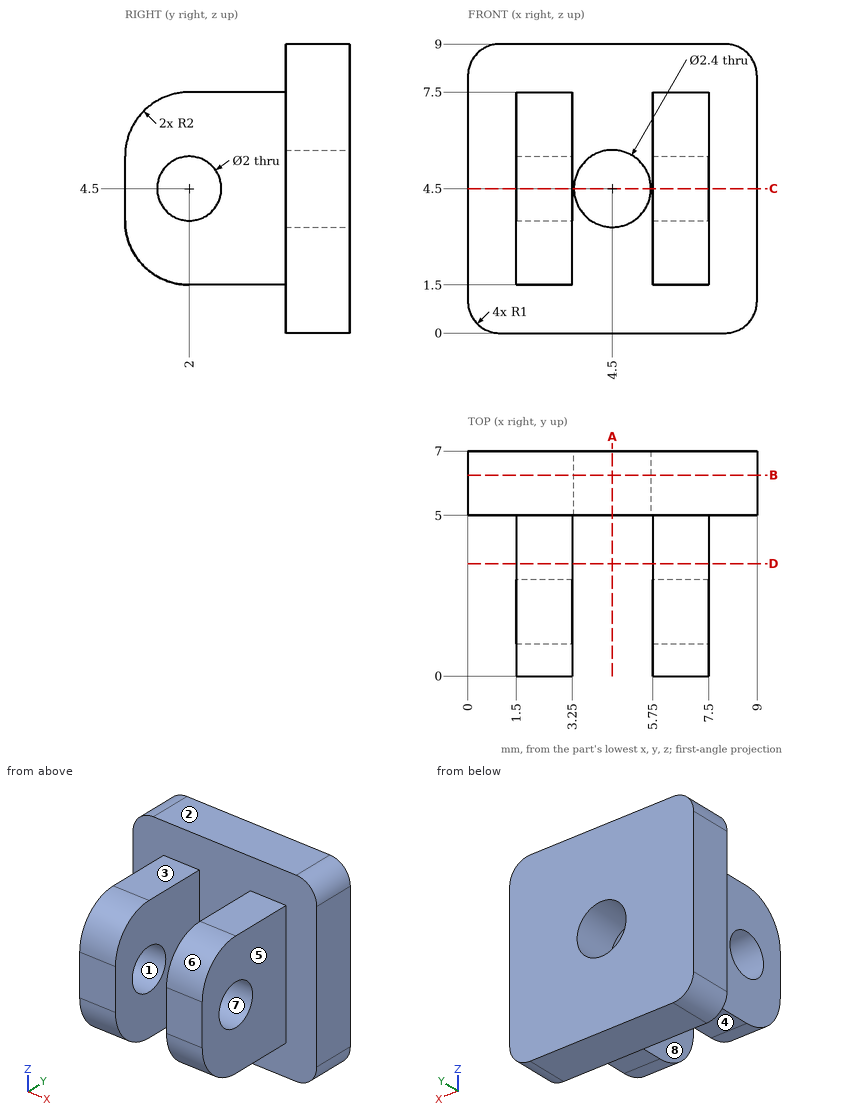
Job drawing, mm, ordinate dimensions from the low corner. One solid piece. A direction names the side the tool comes from. Coordinates: 2 decimals unless noted, no trailing zeros. Order: outer loops, then holes, each group sorted by start corner. A loop starts at its lowest first (then second) coordinate and runs counter-clockwise, first axis right, second up. Notation, with made-up numbers: (19, 21.25) -> (41, 21.25) arc R23 ccw to (41, 41.25) -> close; hole circle Ø11 at (6.25, -3). An arc over 180 degrees is marked (long way). Put each result on its own line as item: value. Start each with the question number.
(1) Pin check, flat tips, straight feed: pin 1 Ø1.9 at (x, y) = (6.5, 3) entering from +Z; pin 2 Ø2.5 at (y, z) = (3, 4) entering from +X; pin 3 Ø1.5 at (y, z) = (3, 4) entering from -X. Stop position of each tip, or through.
(2) Band-saw the part on B-B (y = 6.25). Give the cut face in (x, z).
(3) Band-saw the part on A-A (x = 4.5). Give the cut face in (y, z), then the cut area to 3 significant figures.
(4) Band-saw the part on C-C (z = 4.5). Give the cut face in (x, y), then the cut area to 3 significant figures.
(5) Mould opens along Y. For the marked faces 6, 7 and 8 say: pulls with the +Y half, pulls with the -Y half, needs draft (parallel to the pull), parting line crosses it, or undercut.
(6) Probe line 1 along Z through (x, y) = (2.75, 2); line 2 along X through (y, z) = (3.5, 4.25); line 3 along Z through (x, y) = (4.5, 6.25). List the from-to ranges inside material, lowest first. Write a range as [from, to].
(7) Band-saw the part on D-D (y = 3.5). Give the cut face in (x, z), then the cut area to 3 significant figures.
(8) Which spindle directions (+Z, -Z, +X, -X, +Y, -Y) get a long thin tool onto all of the face, cutting with end or side? Do the marked faces 1, 2, 3, 4 and 5. Say none if no direction does.
Determined:
1. pin 1: stops at z = 7.5
1. pin 2: stops at x = 7.5
1. pin 3: stops at x = 1.5
2. outline: (0, 1) arc R1 ccw to (1, 0) -> (8, 0) arc R1 ccw to (9, 1) -> (9, 8) arc R1 ccw to (8, 9) -> (1, 9) arc R1 ccw to (0, 8) -> close; hole circle Ø2.4 at (4.5, 4.5)
3. outline: (5, 0) -> (7, 0) -> (7, 3.3) -> (5, 3.3) -> close; (5, 5.7) -> (7, 5.7) -> (7, 9) -> (5, 9) -> close
3. area: 13.2 mm²
4. outline: (0, 5) -> (1.5, 5) -> (1.5, 3) -> (3.25, 3) -> (3.25, 5) -> (3.3, 5) -> (3.3, 7) -> (0, 7) -> close; (1.5, 0) -> (3.25, 0) -> (3.25, 1) -> (1.5, 1) -> close; (5.7, 5) -> (5.75, 5) -> (5.75, 3) -> (7.5, 3) -> (7.5, 5) -> (9, 5) -> (9, 7) -> (5.7, 7) -> close; (5.75, 0) -> (7.5, 0) -> (7.5, 1) -> (5.75, 1) -> close
4. area: 23.7 mm²
5. face 6: pulls with the -Y half
5. face 7: undercut
5. face 8: needs draft
6. line 1: z = [1.5, 3.5], [5.5, 7.5]
6. line 2: x = [1.5, 3.25], [5.75, 7.5]
6. line 3: z = [0, 3.3], [5.7, 9]
7. outline: (1.5, 1.5) -> (3.25, 1.5) -> (3.25, 7.5) -> (1.5, 7.5) -> close; (5.75, 1.5) -> (7.5, 1.5) -> (7.5, 7.5) -> (5.75, 7.5) -> close
7. area: 21.0 mm²
8. face 1: +X, -X
8. face 2: +Z, +X, -X, +Y, -Y
8. face 3: +Z, +X, -X, -Y
8. face 4: -Z, +X, -X, -Y
8. face 5: +Z, -Z, +X, -Y
